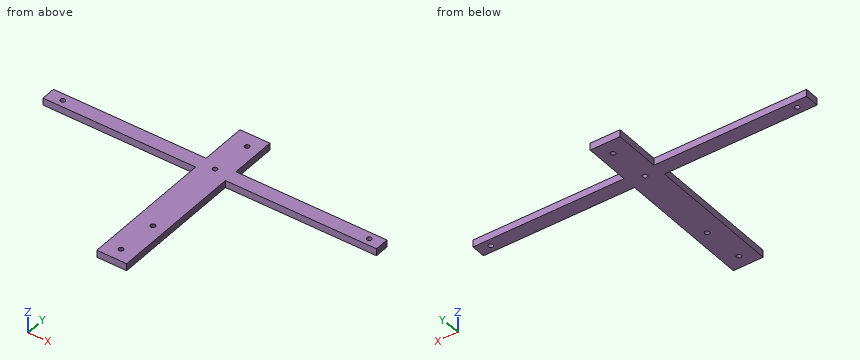
from build123d import *

# Parameters (mm, degrees)
F0_W     = 64.0446986989
F0_H     = 6
F0_R     = 1
F0_W_2   = 63.4251574627
F1_DEPTH = 3


# Not quite as in the source:
# - a feature names something its author has since deleted; it is built from what else it names


with BuildPart() as f1:
    # F0 (on Top) → F1 (new body)
    with BuildSketch(Plane.XY):
        Polygon((-7.5510093011, -42.2321148217), (-1.289947, -42.2321148217), (4.9791345373, -42.2321148217), (4.9791345373, 14.358856), (-1.595708, 14.358856), (-7.5510093011, 14.358856), align=None)
        Polygon((-0.297832, -36.78021), (-0.289947, -36.905543), (-0.297832, -37.030876), (-0.321364, -37.154233), (-0.360171, -37.273667), (-0.41364, -37.387296), (-0.48093, -37.493328), (-0.560978, -37.59009), (-0.652523, -37.676056), (-0.75412, -37.749871), (-0.864168, -37.81037), (-0.98093, -37.856599), (-1.102566, -37.88783), (-1.227157, -37.90357), (-1.352738, -37.90357), (-1.477328, -37.88783), (-1.598964, -37.856599), (-1.715726, -37.81037), (-1.825774, -37.749871), (-1.927371, -37.676056), (-2.018916, -37.59009), (-2.098964, -37.493328), (-2.166254, -37.387296), (-2.219724, -37.273667), (-2.25853, -37.154233), (-2.282062, -37.030876), (-2.289947, -36.905543), (-2.282062, -36.78021), (-2.25853, -36.656853), (-2.219724, -36.537418), (-2.166254, -36.423789), (-2.098964, -36.317758), (-2.018916, -36.220996), (-1.927371, -36.13503), (-1.825774, -36.061215), (-1.715726, -36.000716), (-1.598964, -35.954486), (-1.477328, -35.923256), (-1.352738, -35.907516), (-1.227157, -35.907516), (-1.102566, -35.923256), (-0.98093, -35.954486), (-0.864168, -36.000716), (-0.75412, -36.061215), (-0.652523, -36.13503), (-0.560978, -36.220996), (-0.48093, -36.317758), (-0.41364, -36.423789), (-0.360171, -36.537418), (-0.321364, -36.656853), align=None, mode=Mode.SUBTRACT)
        Polygon((0.834477, -20.078598), (0.842362, -20.203931), (0.834477, -20.329264), (0.810945, -20.452621), (0.772138, -20.572056), (0.718669, -20.685685), (0.651379, -20.791716), (0.571331, -20.888478), (0.479786, -20.974444), (0.378189, -21.048259), (0.268141, -21.108758), (0.151379, -21.154988), (0.029743, -21.186218), (-0.094848, -21.201958), (-0.220429, -21.201958), (-0.345019, -21.186218), (-0.466655, -21.154988), (-0.583417, -21.108758), (-0.693465, -21.048259), (-0.795062, -20.974444), (-0.886607, -20.888478), (-0.966655, -20.791716), (-1.033945, -20.685685), (-1.087415, -20.572056), (-1.126221, -20.452621), (-1.149753, -20.329264), (-1.157638, -20.203931), (-1.149753, -20.078598), (-1.126221, -19.955241), (-1.087415, -19.835807), (-1.033945, -19.722178), (-0.966655, -19.616146), (-0.886607, -19.519384), (-0.795062, -19.433418), (-0.693465, -19.359603), (-0.583417, -19.299104), (-0.466655, -19.252875), (-0.345019, -19.221644), (-0.220429, -19.205904), (-0.094848, -19.205904), (0.029743, -19.221644), (0.151379, -19.252875), (0.268141, -19.299104), (0.378189, -19.359603), (0.479786, -19.433418), (0.571331, -19.519384), (0.651379, -19.616146), (0.718669, -19.722178), (0.772138, -19.835807), (0.810945, -19.955241), align=None, mode=Mode.SUBTRACT)
        Polygon((-7.5510093011, 39.788339287), (-7.5510093011, 20.358856), (-1.595708, 20.358856), (4.9791345373, 20.358856), (4.9791345373, 28.8824737072), (4.9791345373, 39.788339287), (-1.289947, 39.788339287), align=None)
        Polygon((0.834477, 33.921402), (0.842362, 33.796069), (0.834477, 33.670736), (0.810945, 33.547379), (0.772138, 33.427944), (0.718669, 33.314315), (0.651379, 33.208284), (0.571331, 33.111522), (0.479786, 33.025556), (0.378189, 32.951741), (0.268141, 32.891242), (0.151379, 32.845012), (0.029743, 32.813782), (-0.094848, 32.798042), (-0.220429, 32.798042), (-0.345019, 32.813782), (-0.466655, 32.845012), (-0.583417, 32.891242), (-0.693465, 32.951741), (-0.795062, 33.025556), (-0.886607, 33.111522), (-0.966655, 33.208284), (-1.033945, 33.314315), (-1.087415, 33.427944), (-1.126221, 33.547379), (-1.149753, 33.670736), (-1.157638, 33.796069), (-1.149753, 33.921402), (-1.126221, 34.044759), (-1.087415, 34.164193), (-1.033945, 34.277822), (-0.966655, 34.383854), (-0.886607, 34.480616), (-0.795062, 34.566582), (-0.693465, 34.640397), (-0.583417, 34.700896), (-0.466655, 34.747125), (-0.345019, 34.778356), (-0.220429, 34.794096), (-0.094848, 34.794096), (0.029743, 34.778356), (0.151379, 34.747125), (0.268141, 34.700896), (0.378189, 34.640397), (0.479786, 34.566582), (0.571331, 34.480616), (0.651379, 34.383854), (0.718669, 34.277822), (0.772138, 34.164193), (0.810945, 34.044759), align=None, mode=Mode.SUBTRACT)
        with Locations((-39.5733586505, 17.358856)):
            Rectangle(F0_W, F0_H)
        with Locations((-65.4838681221, 17.358856)):
            Circle(F0_R, mode=Mode.SUBTRACT)
        with Locations((36.6917132686, 17.358856)):
            Rectangle(F0_W_2, F0_H)
        with Locations((63.1569251418, 17.358856)):
            Circle(F0_R, mode=Mode.SUBTRACT)
        with BuildLine():
            Line((-7.5510093011, 20.358856), (-7.5510093011, 14.358856))
            Line((-7.5510093011, 14.358856), (-1.595708, 14.358856))
            Line((-1.595708, 14.358856), (-1.595708, 16.358856))
            ThreePointArc((-1.595708, 16.358856), (-2.595708, 17.358856), (-1.595708, 18.358856))
            Line((-1.595708, 18.358856), (-1.595708, 20.358856))
            Line((-1.595708, 20.358856), (-7.5510093011, 20.358856))
        make_face()
        with BuildLine():
            Line((-1.595708, 14.358856), (4.9791345373, 14.358856))
            Line((4.9791345373, 14.358856), (4.9791345373, 20.358856))
            Line((4.9791345373, 20.358856), (-1.595708, 20.358856))
            Line((-1.595708, 20.358856), (-1.595708, 18.358856))
            ThreePointArc((-1.595708, 18.358856), (-0.8886012188, 18.0659627812), (-0.595708, 17.358856))
            ThreePointArc((-0.595708, 17.358856), (-0.8886012188, 16.6517492188), (-1.595708, 16.358856))
            Line((-1.595708, 16.358856), (-1.595708, 14.358856))
        make_face()
    extrude(amount=F1_DEPTH)


solid = f1.part
Verification items for the finished model (mm, model axes). Give positions to 0.01 mm unless a question says otherwise; leave off trailing zeros. Order: outer loops, then holes, each group sorted by start corner. A loop starts at its lowest first (then second) coordinate and runs counter-clockwise, first axis right, second up. Notation, with made-up numbers: M 4.25,79 L 53.25,79 A20 cw 53.25,105 Z; hole C -11,51.25 d10. An arc over 180 degrees is marked long. Answer as a JSON object with one key per item and string values. Group by question number.
1) Cross-section at C-C (y = -5). Enter the section's corners in (x, z), then the cut area to 3 significant figures.
2) Cross-section at B-B (x = -58). Enter the section's corners in (y, z), then the cut area to 3 significant figures.
3) Depth check by flat-ended pin: pin 1 Ø0.9 at (x, z) = (-44.5, 1.5) entering from -Y; pin 2 Ø1.5 at (y, z) = (26, 1) entering from -X; pin 3 Ø1.5 at (y, z) = (-10.5, 1.5) entering from +X. Enter the tip coordinate at first touch or a pass-through.
4) Cross-section at A-A (z = 0.7). Give the number of separate pieces and of enclosed holes in the cut face, then the cut area to 3 significant figures.
5) Scan lines: line 1 along X through (y, z) = (-33, 1.45); line 2 along Y through (x, z) = (18.5, 0.65); line 3 along X through (y, z) = (18, 1). Record each from-to range of solid material in increasing order. Write a range as [from, to].
Result sheet:
{
 "1": {"outline": "M -7.55,0 L 4.98,0 L 4.98,3 L -7.55,3 Z", "area": "37.6 mm2"},
 "2": {"outline": "M 14.36,0 L 20.36,0 L 20.36,3 L 14.36,3 Z", "area": "18.0 mm2"},
 "3": {"pin 1": "stops at y = 14.36", "pin 2": "stops at x = -7.55", "pin 3": "stops at x = 4.98"},
 "4": {"separate pieces": "1", "enclosed holes": "6", "area": "1,770 mm2"},
 "5": {"line 1": "x = [-7.55, 4.98]", "line 2": "y = [14.36, 20.36]", "line 3": "x = [-71.6, -66.25], [-64.72, -2.36], [-0.83, 62.39], [63.92, 68.4]"}
}
